Here's how the part is built. I have some questions about the finished solid (model axes, mm). A direction names the side the tool comes from. Round coordinates to 2 decimals unless told otherwise and drop trailing zeros. Write each loop counter-clockwise with the first axis right and the second up, starting at its lowest first coordinate (ties: lowest second). Pieces come first, ordered by that corner, then holes. Notation, with made-up numbers: (-24.75, -20) -> (-9.75, -20) arc R29 cw to (-9.75, 19) -> close; hole circle Ø10 at (59.5, 78). An arc over 180 degrees is marked (long way). Answer in a Markdown table with one row per item.
from build123d import *

# Parameters (mm, degrees)
SKETCH1_W           = 156
SKETCH1_H           = 85
BOSS_EXTRUDE1_DEPTH = 4
SKETCH2_W           = 15.33
SKETCH2_H           = 4
BOSS_EXTRUDE2_DEPTH = 4
SKETCH3_W           = 31
SKETCH3_H           = 4
CUT_EXTRUDE2_DEPTH  = 4
SKETCH4_W           = 4
SKETCH4_H           = 26.74
SKETCH4_H_2         = 28.24
BOSS_EXTRUDE3_DEPTH = 4
SKETCH5_W           = 10.75
SKETCH5_H           = 4
BOSS_EXTRUDE4_DEPTH = 4
CUT_EXTRUDE3_DEPTH  = 4
SKETCH7_W           = 4
SKETCH7_H           = 8.78
SKETCH7_H_2         = 1.92320958
BOSS_EXTRUDE5_DEPTH = 4
SKETCH8_W           = 4
SKETCH8_H           = 2.999936799
CUT_EXTRUDE4_DEPTH  = 4


with BuildPart() as part:
    # Sketch1 → Boss-Extrude1 (new body)
    with BuildSketch(Plane(origin=(0, 0, 0), x_dir=(1, 0, 0), z_dir=(0, 1, 0))):
        with Locations((78, 42.5)):
            Rectangle(SKETCH1_W, SKETCH1_H)
    extrude(amount=BOSS_EXTRUDE1_DEPTH)

    # Sketch2 → Boss-Extrude2 (add)
    with BuildSketch(Plane(origin=(0, 4, 0), x_dir=(1, 0, 0), z_dir=(0, 1, 0))):
        with Locations((31.495, 87)):
            Rectangle(SKETCH2_W, SKETCH2_H)
        with Locations((74.495, 87)):
            Rectangle(SKETCH2_W, SKETCH2_H)
        with Locations((117.495, 87)):
            Rectangle(SKETCH2_W, SKETCH2_H)
    extrude(amount=-BOSS_EXTRUDE2_DEPTH)

    # Sketch3 → Cut-Extrude2 (cut)
    with BuildSketch(Plane(origin=(0, 4, 0), x_dir=(1, 0, 0), z_dir=(0, 1, 0))):
        with Locations((44, 2)):
            Rectangle(SKETCH3_W, SKETCH3_H)
        with Locations((108, 2)):
            Rectangle(SKETCH3_W, SKETCH3_H)
    extrude(amount=-CUT_EXTRUDE2_DEPTH, mode=Mode.SUBTRACT)

    # Sketch4 → Boss-Extrude3 (add)
    with BuildSketch(Plane(origin=(0, 4, 0), x_dir=(1, 0, 0), z_dir=(0, 1, 0))):
        with Locations((-2, 13.37)):
            Rectangle(SKETCH4_W, SKETCH4_H)
        with Locations((-2, 62.1)):
            Rectangle(SKETCH4_W, SKETCH4_H_2)
    extrude(amount=-BOSS_EXTRUDE3_DEPTH)

    # Sketch5 → Boss-Extrude4 (add)
    with BuildSketch(Plane(origin=(0, 4, 0), x_dir=(1, 0, 0), z_dir=(0, 1, 0))):
        with Locations((144.375, 87)):
            Rectangle(SKETCH5_W, SKETCH5_H)
    extrude(amount=-BOSS_EXTRUDE4_DEPTH)

    # Sketch6 → Cut-Extrude3 (cut)
    with BuildSketch(Plane(origin=(0, 4, 0), x_dir=(1, 0, 0), z_dir=(0, 1, 0))):
        with BuildLine():
            Line((68.5, 22.5), (68.5, 62.5))
            ThreePointArc((68.5, 62.5), (66, 65), (63.5, 62.5))
            Line((63.5, 62.5), (63.5, 22.5))
            ThreePointArc((63.5, 22.5), (66, 20), (68.5, 22.5))
        make_face()
        with BuildLine():
            Line((58.5, 22.5), (58.5, 62.5))
            ThreePointArc((58.5, 62.5), (56, 65), (53.5, 62.5))
            Line((53.5, 62.5), (53.5, 22.5))
            ThreePointArc((53.5, 22.5), (56, 20), (58.5, 22.5))
        make_face()
        with BuildLine():
            Line((78.5, 22.5), (78.5, 62.5))
            ThreePointArc((78.5, 62.5), (76, 65), (73.5, 62.5))
            Line((73.5, 62.5), (73.5, 22.5))
            ThreePointArc((73.5, 22.5), (76, 20), (78.5, 22.5))
        make_face()
        with BuildLine():
            Line((88.5, 22.5), (88.5, 62.5))
            ThreePointArc((88.5, 62.5), (86, 65), (83.5, 62.5))
            Line((83.5, 62.5), (83.5, 22.5))
            ThreePointArc((83.5, 22.5), (86, 20), (88.5, 22.5))
        make_face()
        with BuildLine():
            Line((98.5, 22.5), (98.5, 62.5))
            ThreePointArc((98.5, 62.5), (96, 65), (93.5, 62.5))
            Line((93.5, 62.5), (93.5, 22.5))
            ThreePointArc((93.5, 22.5), (96, 20), (98.5, 22.5))
        make_face()
    extrude(amount=-CUT_EXTRUDE3_DEPTH, mode=Mode.SUBTRACT)

    # Sketch7 → Boss-Extrude5 (add)
    with BuildSketch(Plane(origin=(0, 4, 0), x_dir=(1, 0, 0), z_dir=(0, 1, 0))):
        with Locations((-2, 80.61)):
            Rectangle(SKETCH7_W, SKETCH7_H)
        with Locations((-2, 47.01839521)):
            Rectangle(SKETCH7_W, SKETCH7_H_2)
    extrude(amount=-BOSS_EXTRUDE5_DEPTH)

    # Sketch8 → Cut-Extrude4 (cut)
    with BuildSketch(Plane(origin=(0, 4, 0), x_dir=(1, 0, 0), z_dir=(0, 1, 0))):
        with Locations((-2, 25.240031601)):
            Rectangle(SKETCH8_W, SKETCH8_H)
    extrude(amount=-CUT_EXTRUDE4_DEPTH, mode=Mode.SUBTRACT)


solid = part.part
1) I want a section at C-C, the plane z = -26.5. List the corners of the cut face in (x, y) for me, and give its area (3 significant figures).
Response:
| item | result |
|---|---|
| outline | (0, 0) -> (53.5, 0) -> (53.5, 4) -> (0, 4) -> close; (58.5, 0) -> (63.5, 0) -> (63.5, 4) -> (58.5, 4) -> close; (68.5, 0) -> (73.5, 0) -> (73.5, 4) -> (68.5, 4) -> close; (78.5, 0) -> (83.5, 0) -> (83.5, 4) -> (78.5, 4) -> close; (88.5, 0) -> (93.5, 0) -> (93.5, 4) -> (88.5, 4) -> close; (98.5, 0) -> (156, 0) -> (156, 4) -> (98.5, 4) -> close |
| area | 524 mm^2 |
2) I want a section at B-B, the plane z = -51.5. List the corners of the cut face in (x, y) for me.
Response:
| item | result |
|---|---|
| outline | (-4, 0) -> (53.5, 0) -> (53.5, 4) -> (-4, 4) -> close; (58.5, 0) -> (63.5, 0) -> (63.5, 4) -> (58.5, 4) -> close; (68.5, 0) -> (73.5, 0) -> (73.5, 4) -> (68.5, 4) -> close; (78.5, 0) -> (83.5, 0) -> (83.5, 4) -> (78.5, 4) -> close; (88.5, 0) -> (93.5, 0) -> (93.5, 4) -> (88.5, 4) -> close; (98.5, 0) -> (156, 0) -> (156, 4) -> (98.5, 4) -> close |
3) For pin 1 (1.2 mm diameter, centred on y = 2.5, z = -87, fed in from +X); pin 2 (1.2 mm diameter, centred on x = 133.5, y = 2, fed in from -Z); pin 3 (2 mm diameter, centred on x = 49.5, y = 1, fed in from +Z); pin 4 (1.5 mm diameter, centred on x = 97.5, z = -54, fed in from -Y), each with a flat end and sliding along its axis, tell me the tip position at first contact or that it passes through.
Response:
| item | result |
|---|---|
| pin 1 | stops at x = 149.75 |
| pin 2 | stops at z = -85 |
| pin 3 | stops at z = -4 |
| pin 4 | passes through |
4) Which directions (+Z, -Z, +X, -X, +Y, -Y) give clear straight access to the entire face, cutting with the end or side of a thin tool? Please do faces 1 (the face through (0, 2, -35)), 2 (the face through (82.16, 2, -87)), 3 (the face through (123.5, 2, -2)), 4 (the face through (66, 2, -65)), 5 (the face through (23.83, 2, -87)).
Response:
| item | result |
|---|---|
| face 1 | -X, +Y, -Y |
| face 2 | -Z, +Y, -Y |
| face 3 | +Z, +Y, -Y |
| face 4 | +Y, -Y |
| face 5 | -Z, -X, +Y, -Y |
5) I want a section at D-D, the plane x = 96. List the corners of the cut face in (y, z) for me.
Response:
| item | result |
|---|---|
| outline | (0, -85) -> (4, -85) -> (4, -65) -> (0, -65) -> close; (0, -20) -> (4, -20) -> (4, -4) -> (0, -4) -> close |
6) I want a section at A-A, the plane x = 76. List the corners of the cut face in (y, z) for me.
Response:
| item | result |
|---|---|
| outline | (0, -89) -> (4, -89) -> (4, -65) -> (0, -65) -> close; (0, -20) -> (4, -20) -> (4, 0) -> (0, 0) -> close |
7) I need wall thicknesses on line 1 (X direction, y = 1.55, z = -59.5); line 2 (X direction, y = 3.2, z = -25); line 3 (Z direction, x = 93, y = 2.6). Which ranges of each line are inside material? Lowest first, please. Write a range as [from, to].
Response:
| item | result |
|---|---|
| line 1 | x = [-4, 53.5], [58.5, 63.5], [68.5, 73.5], [78.5, 83.5], [88.5, 93.5], [98.5, 156] |
| line 2 | x = [0, 53.5], [58.5, 63.5], [68.5, 73.5], [78.5, 83.5], [88.5, 93.5], [98.5, 156] |
| line 3 | z = [-85, -4] |
8) We'd pull the mould along X, two halves only. Please class faces 6 (the face through (156, 2, -42)), 7 (the face through (76, 2, -20)), 8 (the face through (-4, 2, -65)), 9 (the face through (93, 0, -45)): +X half, -X half, draft (parallel to the pull), parting line (faces both ways), or undercut.
Response:
| item | result |
|---|---|
| face 6 | +X half |
| face 7 | undercut |
| face 8 | -X half |
| face 9 | draft |
